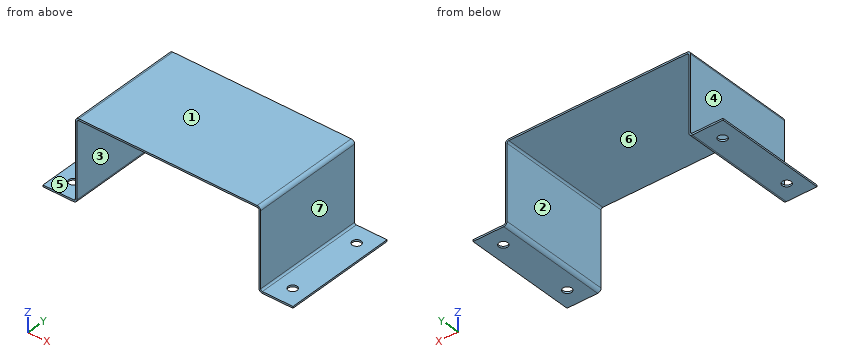
Autodesk Inventor part; units mm, degrees
ref_plane "YZ Plane" through (0, 0, 0) normal (1, 0, 0) x (0, 1, 0)
ref_plane "XZ Plane" through (0, 0, 0) normal (0, 1, 0) x (-1, 0, 0)
ref_plane "XY Plane" through (0, 0, 0) normal (0, 0, 1) x (1, 0, 0)
sketch "Boceto1" plane through (0, 0, 0) normal (0, 0, 1) x (1, 0, 0)
  line L0 (0, 0) -> (80, 0)
  line L1 (80, 0) -> (80, 50)
  line L2 (80, 50) -> (0, 50)
  line L3 (0, 50) -> (0, 0)
  dimension "d0" = 80
  dimension "d1" = 50
extrude "Placa1" add sketch "Boceto1" along normal blind 0.76
sketch "Boceto2" plane through (80, 50, 0) normal (1, 0, 0) x (0, 1, 0)
  line L0 (-50, 0) -> (0, 0)
  line L1 (0, 0) -> (0, 34.24)
  line L2 (0, 34.24) -> (-50, 34.24)
  line L3 (-50, 34.24) -> (-50, 0)
edge flange "Pestaña1" height 35 angle 90 thickness 0.76 bend radius 0.76 thickness toward (1, 0, 0) relief tear relief width 0.76 relief depth 0.38 corner gap 0.76 corner form 0 edges at (80, 25, 0.76) (0, 25, 0.76) wall of the first edge with corners at (80, 0, 0) (80, 50, 0) (80, 50, -34.24) (80, 0, -34.24)
bend "Doblez1"
corner "Esquina1"
sketch "Boceto3" plane through (-0.76, 50, -34.24) normal (0, 0, -1) x (1, 0, 0)
  line L0 (0, -50) -> (0, 0)
  line L1 (0, 0) -> (-14.24, 0)
  line L2 (-14.24, 0) -> (-14.24, -50)
  line L3 (-14.24, -50) -> (0, -50)
edge flange "Pestaña2" height 15 angle 90 thickness 0.76 bend radius 0.76 thickness toward (0, 0, -1) relief tear relief width 0.76 relief depth 0.38 corner gap 0.76 corner form 0 edges at (0, 25, -34.24) (80, 25, -34.24) wall of the first edge with corners at (-0.76, 0, -34.24) (-0.76, 50, -34.24) (-15, 50, -34.24) (-15, 0, -34.24)
bend "Doblez2"
corner "Esquina2"
sketch "Boceto4" plane through (-15, 0, -35) normal (0, 0, -1) x (-1, 0, 0)
  circle A0 centre (-6.74, 8) radius 1.95
  circle A1 centre (-6.74, 42) radius 1.95
  point P0 (-15, 0)
  dimension "d23" = 3.9
  dimension "d24" = 3.9
extrude "Extrusión1" cut sketch "Boceto4" against normal through all
sketch "Boceto5" plane through (95, 0, -35) normal (0, 0, -1) x (-1, 0, 0)
  circle A0 centre (6.74, 8) radius 1.95
  circle A1 centre (6.74, 42) radius 1.95
  point P0 (95, 0)
  dimension "d27" = 3.9
  dimension "d28" = 3.9
extrude "Extrusión2" cut sketch "Boceto5" against normal through all
sketch "Boceto6" plane through (0, 0, 0.76) normal (0, 0, 1) x (1, 0, 0)
  point P0 (0, 0)
equation "\"d24\" = d23"
equation "\"d28\" = d27"
equation "\"d2\" = Grosor"
equation "\"d3\" = Anchura_desahogo_plegado"
equation "\"d4\" = Profundidad_desahogo_plegado"
equation "\"d5\" = Remanente_mínimo"
equation "\"d6\" = Radiodetransición"
equation "\"d9\" = Radio_pliegue"
equation "\"d10\" = Tamaño_destalonado"
equation "\"d11\" = TamañoSeparación"
equation "\"d12\" = Tamaño_de_radio_de_Jacobi"
equation "\"d13\" = Anchura_desahogo_plegado"
equation "\"d14\" = Profundidad_desahogo_plegado"
equation "\"d15\" = Remanente_mínimo"
equation "\"d16\" = Radiodetransición"
equation "\"d19\" = Radio_pliegue"
equation "\"d20\" = Tamaño_destalonado"
equation "\"d21\" = TamañoSeparación"
equation "\"d22\" = Tamaño_de_radio_de_Jacobi"
equation "\"Radio_pliegue\" = Grosor"
equation "\"Anchura_desahogo_plegado\" = Grosor"
equation "\"Profundidad_desahogo_plegado\" = 0.5 * Grosor"
equation "\"Tamaño_destalonado\" = 4 * Grosor"
equation "\"Remanente_mínimo\" = 2 * Grosor"
equation "\"Radiodetransición\" = Radio_pliegue"
equation "\"Tamaño_de_radio_de_Jacobi\" = Radio_pliegue"
equation "\"TamañoSeparación\" = Grosor"
properties part number "Base Valvula" material "Steel AISI 1006 85 HR"
Geometry: final body of the model. Coordinates: model frame, mm. Face numbers are marked on the shaded views. A direction names the side the tool comes from. Coordinates: 2 decimals unless noted, no trailing zeros. Loops run counter-clockwise (first coordinate to the right, second up) from the corner with the lowest first, then second, coordinate; pieces in that order, holes last. Notation, with made-up numbers: (73, 77.5) - (132, 77.5) arc R15 ccw to (132, 96.5) - close; hole circle Ø4 at (10.5, 19.5). An arc over 180 degrees is marked (long way). One line per question, with ' | ' between items. Start each with the question number.
(1) Ray query, L1, parallel to Y at x = 88.26, z = -34.6; L2, parallel to X at y = 19.5, z = -21.5; L3, parallel to Z at x = 44.5, y = 47. Return the intervals inside material, ascending. Write a range as from..to.
(2) Cut plane D-D on x = 73.5. Output: boundary loops of the cut face in (y, z), and give its area (3 significant figures).
(3) Draft query along X for the marked faces 1, 2, 3 and 4. Return one class per face: +X half, -X half, draft (parallel to the pull), parting line (faces both ways), or undercut.
(4) First-contact query: pin 1 (4.5 mm diameter, centred on x = 88.26, y = 8, fed in from +Z); pin 2 (2 mm diameter, centred on y = 36, z = -27.5, fed in from +X); pin 3 (1 mm diameter, centred on y = 23.5, z = -29.5, fed in from -X). Flat tips, straight axial feed; report the tip coordinate or a pass-through.
(5) Cut plane A-A on x = 88.26. Output: boundary loops of the cut face in (y, z).
(6) Cut plane C-C on z = -26. Output: boundary loops of the cut face in (x, y), and give its area (3 significant figures).
(7) Cut plane B-B on y = 8. Output: boundary loops of the cut face in (x, z).
(8) Reachability of the marked faces 5, 6 and 7 from +Z, -Z, +X, -X, +Y, -Y: full face, straight path, thin tool, end or side. Return the list, or none.
Here are the results:
1) L1: 0..6.05, 9.95..40.05, 43.95..50 | L2: -0.76..0, 80..80.76 | L3: 0..0.76
2) outline: (0, 0) - (50, 0) - (50, 0.76) - (0, 0.76) - close | area: 38.0 mm²
3) face 1: draft | face 2: undercut | face 3: undercut | face 4: -X half
4) pin 1: z = -34.24 | pin 2: x = 80.76 | pin 3: x = -0.76
5) outline: (0, -35) - (6.05, -35) - (6.05, -34.24) - (0, -34.24) - close; (9.95, -35) - (40.05, -35) - (40.05, -34.24) - (9.95, -34.24) - close; (43.95, -35) - (50, -35) - (50, -34.24) - (43.95, -34.24) - close
6) outline: (-0.76, 0) - (0, 0) - (0, 50) - (-0.76, 50) - close; (80, 0) - (80.76, 0) - (80.76, 50) - (80, 50) - close | area: 76.0 mm²
7) outline: (-15, -35) - (-10.21, -35) - (-10.21, -34.24) - (-15, -34.24) - close; (-6.31, -35) - (-1.52, -35) arc R1.52 ccw to (0, -33.48) - (0, -0.76) arc R0.76 cw to (0.76, 0) - (79.24, 0) arc R0.76 cw to (80, -0.76) - (80, -33.48) arc R1.52 ccw to (81.52, -35) - (86.31, -35) - (86.31, -34.24) - (81.52, -34.24) arc R0.76 cw to (80.76, -33.48) - (80.76, -0.76) arc R1.52 ccw to (79.24, 0.76) - (0.76, 0.76) arc R1.52 ccw to (-0.76, -0.76) - (-0.76, -33.48) arc R0.76 cw to (-1.52, -34.24) - (-6.31, -34.24) - close; (90.21, -35) - (95, -35) - (95, -34.24) - (90.21, -34.24) - close
8) face 5: +Z, -X, +Y, -Y | face 6: -Z, +Y, -Y | face 7: +Z, +X, +Y, -Y
